Verification items for the finished model (mm, model axes). A direction names the side the tool comes from. Give positions to 0.01 mm unless a question says otherwise; leave off trailing zeros. Order: outer loops, then holes, each group sorted by start corner. A loop starts at its lowest first (then second) coordinate and runs counter-clockwise, first axis right, second up. Notation, with made-up numbers: (84, -16) - (104, -16) arc R24 cw to (104, -2) - close; hole circle Ø6 at (-31.75, 59.5). An arc over 180 degrees is marked (long way). Answer as a JSON object with one key per item and string values. Group by question number.
(1) Depth check by flat-ended pin: pin 1 Ø8.5 at (y, z) = (15.5, 17.5) entering from -X; pin 2 Ø2.5 at (x, z) = (-17.05, 17.1) entering from +Y; pin 3 Ø2.5 at (x, z) = (-13.5, 7) entering from +Y. Enter the tip coordinate at first touch or a pass-through.
(2) Access from +Z, -Z, +X, -X, +Y, -Y to the whole of each face (thin tool, end or side, straight path). Record for faces 1 (the face through (-67.95, 16.88, 2.57)), 2 (the face through (-17, 31.2, 19)), 3 (the face through (-17.41, 31.84, 15.49)), 4 (the face through (-0.43, 17.32, 33.75)).
(3) Thickness scan on line 1 (Y direction, x = -51.5, z = 28); line 2 (X direction, y = 21, z = 25); line 3 (Y direction, x = -34, z = 17). Record the ranges inside material, lowest first.
(4) Section check C-C (x = -39). Record the boundary of the cut face in (y, z).
(5) Mould release check, pull along Y, two halves, no side actions. Record for faces 5 (the face through (-52, 17, 31.2)), 6 (the face through (-34, 0, 17)), 7 (the face through (-0.45, 17.32, 0.43)): +Y half, -Y half, draft (parallel to the pull), parting line (faces both ways), or undercut.
```python
from build123d import *

# Parameters (mm, degrees)
F1_DEPTH              = 34.2
F2_W                  = 28.2
F2_H                  = 28.2
F3_DEPTH              = 31.2
F4_W                  = 34.2
F4_H                  = 34.2
F5_DEPTH              = 34.2
F6_W                  = 28.2
F6_H                  = 28.2
F7_DEPTH              = 31.2
F10_D                 = 3.3
F10_DEPTH             = 25
F10_CSINK_D           = 6.72
F10_CSINK_ANGLE       = 90
F10_TIP               = 0.9914200214
F10_ON_F9_D           = 3.3
F10_ON_F9_DEPTH       = 25
F10_ON_F9_CSINK_D     = 6.72
F10_ON_F9_CSINK_ANGLE = 90
F10_ON_F9_TIP         = 0.9914200214
F11_R                 = 1.49999
F12_W                 = 5
F12_H                 = 5
F13_DEPTH             = 2.5


# Not quite as in the source:
# - a fillet or chamfer is up to 0.001 mm smaller than in the source, because OpenCascade refuses the exact size
# - a feature names something its author has since deleted; it is built from what else it names


with BuildPart() as f1:
    # F0 (on Top) → F1 (new body)
    with BuildSketch(Plane.XY):
        Polygon((-34.2, 0), (-8, 0), (0, 0), (0, 34.2), (-34.2, 34.2), align=None)
    extrude(amount=F1_DEPTH)

    # F2 (on face) → F3 (cut)
    with BuildSketch(Plane.XY.offset(34.2)):
        with Locations((-17.1, 17.1)):
            Rectangle(F2_W, F2_H)
    extrude(amount=-F3_DEPTH, mode=Mode.SUBTRACT)

    # F4 (on face) → F5 (join)
    with BuildSketch(Plane(origin=(-34.2, 0, 0), x_dir=(0, -1, 0), z_dir=(-1, 0, 0))):
        with Locations((-17.1, 17.1)):
            Rectangle(F4_W, F4_H)
    extrude(amount=F5_DEPTH)

    # F6 (on face) → F7 (cut)
    with BuildSketch(Plane(origin=(-68.4, 0, 0), x_dir=(0, -1, 0), z_dir=(-1, 0, 0))):
        with Locations((-17.1, 17.1)):
            Rectangle(F6_W, F6_H)
    extrude(amount=-F7_DEPTH, mode=Mode.SUBTRACT)

    # F10
    with Locations(Plane(origin=(0, 34.2, 0), x_dir=(-1, 0, 0), z_dir=(0, 1, 0))):
        with Locations((17.05, 17.1), (51.35, 17.1)):
            CounterSinkHole(F10_D / 2, F10_CSINK_D / 2, depth=F10_DEPTH, counter_sink_angle=F10_CSINK_ANGLE)
            with Locations((0, 0, -(F10_DEPTH + F10_TIP / 2))):  # 118° drill point
                Cone(0, F10_D / 2, F10_TIP, mode=Mode.SUBTRACT)

    # F10 on F9
    with Locations(Plane(origin=(-37.2, 0, 0), x_dir=(0, -1, 0), z_dir=(-1, 0, 0))):
        with Locations((-17.1, 17.1)):
            CounterSinkHole(F10_ON_F9_D / 2, F10_ON_F9_CSINK_D / 2, depth=F10_ON_F9_DEPTH, counter_sink_angle=F10_ON_F9_CSINK_ANGLE)
            with Locations((0, 0, -(F10_ON_F9_DEPTH + F10_ON_F9_TIP / 2))):  # 118° drill point
                Cone(0, F10_ON_F9_D / 2, F10_ON_F9_TIP, mode=Mode.SUBTRACT)

    # F11 (radius 1.5 in the source; OpenCascade refuses exactly that, so slightly less here)
    f11_edges = [f1.edges().sort_by_distance(p)[0] for p in [
        (-31.2, 17.1, 34.2),
        (-17.1, 31.2, 34.2),
        (-17.1, 31.2, 3),
        (0, 17.1, 34.2),
        (-34.2, 0, 34.2),
        (-68.4, 17.1, 34.2),
        (-34.2, 34.2, 34.2),
        (0, 34.2, 17.1),
        (-68.4, 17.1, 31.2),
        (-68.4, 0, 17.1),
        (-68.4, 3, 17.1),
        (-68.4, 31.2, 17.1),
        (-68.4, 34.2, 17.1),
        (-68.4, 17.1, 3),
        (-68.4, 17.1, 0),
        (-34.2, 0, 0),
        (-34.2, 34.2, 0),
        (0, 0, 17.1),
        (-3, 17.1, 34.2),
        (-17.1, 3, 34.2),
        (0, 17.1, 0),
    ]]
    fillet(f11_edges, radius=F11_R)

    # F12 (on face) → F13 (cut)
    with BuildSketch(Plane(origin=(0, 34.2, 0), x_dir=(-1, 0, 0), z_dir=(0, 1, 0))):
        with Locations((14.6, 6.5)):
            Rectangle(F12_W, F12_H)
    extrude(amount=-F13_DEPTH, mode=Mode.SUBTRACT)


solid = f1.part
```
Solutions:
{
 "1": {"pin 1": "stops at x = -37.2", "pin 2": "stops at y = 3", "pin 3": "stops at y = 31.7"},
 "2": {"face 1": "-X", "face 2": "+Z", "face 3": "+Y", "face 4": "+Z, +X, +Y, -Y"},
 "3": {"line 1": "y = 0 to 3, 31.2 to 34.2", "line 2": "x = -37.2 to -31.2, -3 to 0", "line 3": "y = 0 to 15.45, 18.75 to 34.2"},
 "4": {"outline": "(0, 1.5) arc R1.5 ccw to (1.5, 0) - (32.7, 0) arc R1.5 ccw to (34.2, 1.5) - (34.2, 32.7) arc R1.5 ccw to (32.7, 34.2) - (1.5, 34.2) arc R1.5 ccw to (0, 32.7) - close; hole (3, 3) - (31.2, 3) - (31.2, 31.2) - (3, 31.2) - close"},
 "5": {"face 5": "undercut", "face 6": "-Y half", "face 7": "draft"}
}
